```python
from build123d import *

# Parameters (mm, degrees)
SKE1_R          = 3.91
BASE1_DEPTH     = 4.78
BODYSKE_W       = 20.66
BODYSKE_H       = 2.39
HEX_2_DEPTH     = 1.3
SKE9_R          = 2.5
CHAMFER_2_DEPTH = 1.3
CHAMFER_2_DRAFT = -60
CHAMFER1_SIZE   = 0.5


with BuildPart() as part:
    # Ske1 → Base1 (new body)
    with BuildSketch(Plane.XY):
        Circle(SKE1_R)
    extrude(amount=BASE1_DEPTH)

    # BodySke → BaseBody (revolve)
    with BuildSketch(Plane(origin=(0, 0, 0), x_dir=(0, 0, -1), z_dir=(1, 0, 0)), mode=Mode.PRIVATE) as basebody_sk:
        with Locations((5.55, 1.195)):
            Rectangle(BODYSKE_W, BODYSKE_H)
    revolve(basebody_sk.sketch.rotate(Axis((0, 0, 1.385793675), (0, 0, -1)), 90), axis=Axis((0, 0, 1.385793675), (0, 0, -1)))

    # Ske8 → Hex 2 (cut)
    with BuildSketch(Plane.XY.offset(4.78)):
        Polygon((0, 2.292080569), (-1.985, 1.146040284), (-1.985, -1.146040284), (0, -2.292080569), (1.985, -1.146040284), (1.985, 1.146040284), align=None)
    extrude(amount=-HEX_2_DEPTH, mode=Mode.SUBTRACT)


with BuildPart() as chamfer_2_tool:
    # Ske9 → Chamfer 2 (with draft: the straight prism first)
    with BuildSketch(Plane.XY.offset(4.78)):
        Circle(SKE9_R)
    extrude(amount=-CHAMFER_2_DEPTH)
    # Chamfer 2: the draft: its side faces are tilted about the plane it starts from
    chamfer_2_sides = [chamfer_2_tool.faces().sort_by_distance(p)[0] for p in [
        (-2.5, 0, 4.13),
    ]]
    draft(chamfer_2_sides, Plane.XY.offset(4.78), CHAMFER_2_DRAFT)


with BuildPart() as part_1:
    add(part.part)

    # Chamfer 2: cut by chamfer_2_tool
    add(chamfer_2_tool.part, mode=Mode.SUBTRACT)

    # Chamfer1
    chamfer1_edges = [part_1.edges().sort_by_distance(p)[0] for p in [
        (-3.91, 0, 4.78),
        (-2.39, 0, -15.88),
    ]]
    chamfer(chamfer1_edges, length=CHAMFER1_SIZE)


solid = part_1.part
```
For this review, take the finished solid that the model builds, in its own axes (mm). A direction names the side the tool comes from. Give positions to 0.01 mm unless a question says otherwise; leave off trailing zeros. Write each loop counter-clockwise with the first axis right and the second up, starting at its lowest first coordinate (ties: lowest second). Pieces come first, ordered by that corner, then holes. Notation, with made-up numbers: M -14.5,83.25 L 26.5,83.25 A15 ccw 26.5,96.25 Z; hole C -26.75,78.5 d1. An arc over 180 degrees is marked long. Answer as a JSON object with one key per item and string values. Group by question number.
Item 1: Consider section B-B on z = 0.25. Write out the cut boundary in (x, y).
Item 2: Consider section C-C on z = -12. Write out the cut boundary in (x, y).
Item 3: Tool access review of faces 1 (the cylindrical face through (2.28, -0.72, -7.8)), 2 (the flat face through (-1.01, -1.71, 4.08)), 3 (the flat face through (2, -2, 4.78)): name each direction out of +Z, -Z, +X, -X, +Y, -Y from which nothing blocks a thin tool from reaching the whole face with its end or side.
Item 4: For pin 1 Ø1 at (x, y) = (2, 2) entering from -Z; pin 2 Ø0.9 at (y, z) = (0.5, 4) entering from -X; pin 3 Ø3 at (x, y) = (0, 0.5) entering from +Z, all flat-tipped, find the tip position at first contact; note any pin that passes through.
Item 5: For probe 1 along Z at (x, y) = (3, 1); probe 2 along Y at (x, z) = (0, -10.25); probe 3 along Z at (x, y) = (-1, 0.5), list the stretches that pass through material, from the lowest coordinate up. Write a range as [from, to].
Item 6: Consider section A-A on y = 0. Write out the cut boundary in (x, z) (3 decimals), plus the area to 3 significant figures.
Item 7: Draft analysis for pull direction X (two halves, no side actions). For faces 4 (the cylindrical face through (3.73, 1.17, 2.11)), 5 (the flat face through (1.985, 0, 4)), 6 (the flat face through (-2, -2, 0)), state which applies: +X half, -X half, draft (parallel to the pull), parting line (faces both ways), or undercut.
Check result:
{
 "1": {"outline": "C 0,0 d7.82"},
 "2": {"outline": "C 0,0 d4.78"},
 "3": {"face 1": "-Z", "face 2": "+Z", "face 3": "+Z, +X, -X, +Y, -Y"},
 "4": {"pin 1": "stops at z = -15.44", "pin 2": "stops at x = -3.91", "pin 3": "stops at z = 3.48"},
 "5": {"probe 1": "z = [0, 4.78]", "probe 2": "y = [-2.39, 2.39]", "probe 3": "z = [-15.88, 3.48]"},
 "6": {"outline": "M -3.91,0 L -2.39,0 L -2.39,-15.38 L -1.89,-15.88 L 1.89,-15.88 L 2.39,-15.38 L 2.39,0 L 3.91,0 L 3.91,4.28 L 3.41,4.78 L 2.5,4.78 L 1.985,4.483 L 1.985,3.48 L -1.985,3.48 L -1.985,4.483 L -2.5,4.78 L -3.41,4.78 L -3.91,4.28 Z", "area": "107 mm^2"},
 "7": {"face 4": "parting line", "face 5": "undercut", "face 6": "draft"}
}
